Part model, mm, in its own coordinate system. Round coordinates to 2 decimals unless told otherwise and drop trailing zeros. Write each loop counter-clockwise with the first axis right and the second up, starting at its lowest first coordinate (ties: lowest second). Pieces come first, ordered by that corner, then holes. Notation, with made-up numbers: (-31, 72.5) -> (16, 72.5) arc R33 cw to (16, 100.5) -> close; hole circle Ø2 at (-0.5, 54). An arc over 180 degrees is marked (long way). Return JSON: item names as keys, results as strings. Group by question number.
(1) Saw through at B-B (z = 42.5). List the corners of the cut face in (x, y), plus the area to 3 significant figures.
(2) Drop flat-ended pins along their axis: pin 1 Ø0.8 at (x, y) = (2.5, 4) entering from +Z; pin 2 Ø2 at (y, z) = (3, 40.5) entering from +X; pin 3 Ø24 at (x, z) = (37, 57.5) entering from +Y. Give the stop position or say it passes through.
(3) Saw through at D-D (z = 18). List the corners of the cut face in (x, y).
(4) Drill centre lines: L1, parallel to X at y = 3.5, z = 37.5; L2, parallel to Y at x = 69, z = 30; L3, parallel to X at y = 6.25, z = 35. Where is each one in solid material? Low to high. Write a range as from..to.
(5) Saw through at A-A (y = 4). List the corners of the cut face in (x, z).
(6) Saw through at C-C (x = 96.5). List the corners of the cut face in (y, z), plus the area to 3 significant figures.
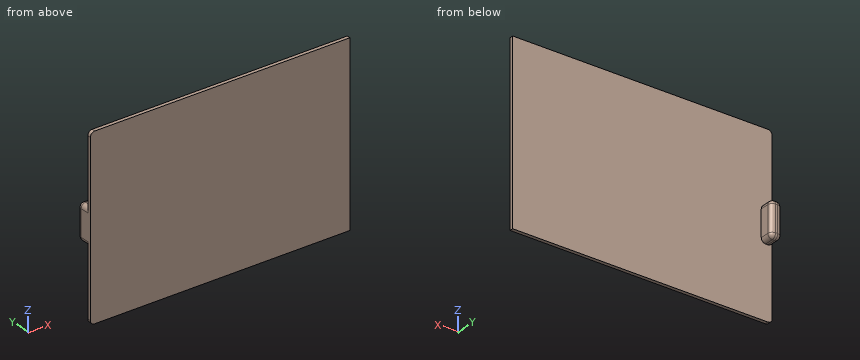
from build123d import *

# Parameters (mm, degrees)
SKETCH1_W           = 118
SKETCH1_H           = 80.5
LID_EXTRUDE_DEPTH   = 1.6
LID_EDGE_FILLET_R   = 2
SKETCH2_W           = 5
SKETCH2_H           = 16
BOSS_EXTRUDE2_DEPTH = 6
FILLET2_R           = 2


with BuildPart() as part:
    # Sketch1 → lid extrude (new body)
    with BuildSketch(Plane(origin=(0, 0, 0), x_dir=(1, 0, 0), z_dir=(0, 1, 0))):
        with Locations((59, -40.25)):
            Rectangle(SKETCH1_W, SKETCH1_H)
    extrude(amount=LID_EXTRUDE_DEPTH)

    # lid edge fillet
    lid_edge_fillet_edges = [part.edges().sort_by_distance(p)[0] for p in [
        (0, 0.8, 0),
        (0, 0.8, 80.5),
    ]]
    fillet(lid_edge_fillet_edges, radius=LID_EDGE_FILLET_R)

    # Sketch2 → Boss-Extrude2 (add)
    with BuildSketch(Plane(origin=(0, 1.6, 0), x_dir=(1, 0, 0), z_dir=(0, 1, 0))):
        with Locations((2.5, -40.25)):
            Rectangle(SKETCH2_W, SKETCH2_H)
    extrude(amount=BOSS_EXTRUDE2_DEPTH)

    # Fillet2
    fillet2_edges = [part.edges().sort_by_distance(p)[0] for p in [
        (0, 4.6, 32.25),
        (2.5, 7.6, 48.25),
        (0, 4.6, 48.25),
        (5, 7.6, 40.25),
        (5, 4.6, 48.25),
        (2.5, 7.6, 32.25),
        (5, 4.6, 32.25),
        (0, 7.6, 40.25),
    ]]
    fillet(fillet2_edges, radius=FILLET2_R)


solid = part.part
Computed values:
{
 "1": {"outline": "(0, 0) -> (118, 0) -> (118, 1.6) -> (5, 1.6) -> (5, 5.6) arc R2 ccw to (3, 7.6) -> (2, 7.6) arc R2 ccw to (0, 5.6) -> close", "area": "217 mm2"},
 "2": {"pin 1": "z = 48.25", "pin 2": "x = 5", "pin 3": "y = 1.6"},
 "3": {"outline": "(0, 0) -> (118, 0) -> (118, 1.6) -> (0, 1.6) -> close"},
 "4": {"L1": "0..5", "L2": "0..1.6", "L3": "0.11..4.89"},
 "5": {"outline": "(0, 34.25) arc R2 ccw to (2, 32.25) -> (3, 32.25) arc R2 ccw to (5, 34.25) -> (5, 46.25) arc R2 ccw to (3, 48.25) -> (2, 48.25) arc R2 ccw to (0, 46.25) -> close"},
 "6": {"outline": "(0, 0) -> (1.6, 0) -> (1.6, 80.5) -> (0, 80.5) -> close", "area": "129 mm2"}
}
